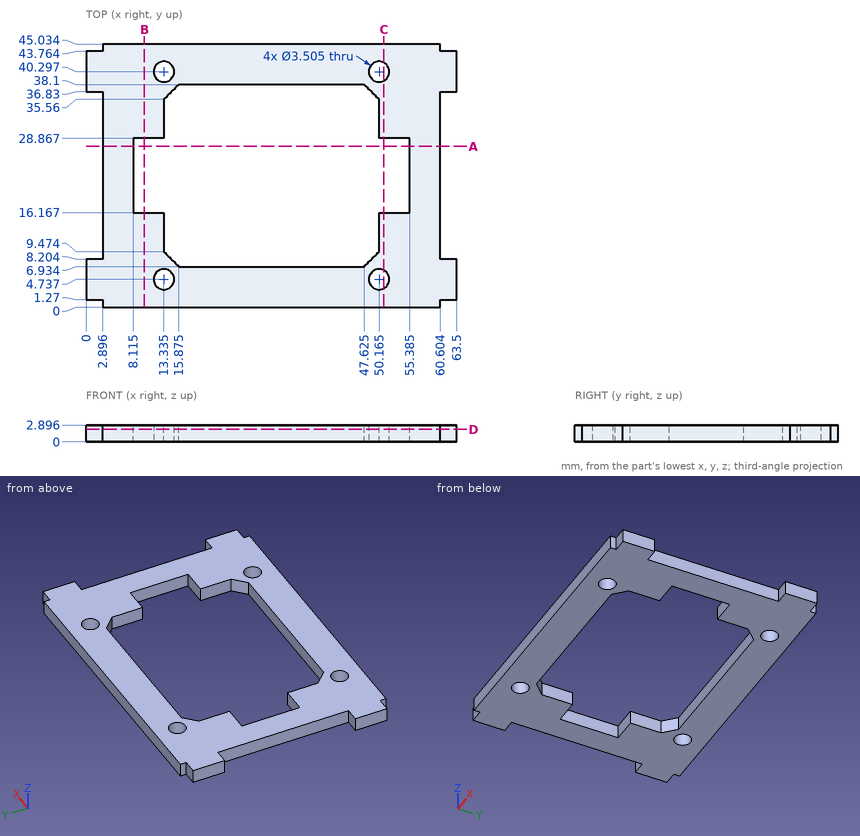
Job drawing, mm, ordinate dimensions from the low corner. One solid piece. Give positions to 0.01 mm unless a question says otherwise; leave off trailing zeros. Order: outer loops, then holes, each group sorted by start corner. A loop starts at its lowest first (then second) coordinate and runs counter-clockwise, first axis right, second up. Notation, with made-up numbers: M 63,4 L 89,4 A34 ccw 89,37 Z; hole C 25.25,26.5 d11. An arc over 180 degrees is marked long. Return JSON: item names as keys, results as strings.
Q1. Band-saw the part on D-D (z = 2.15). Count the separate pieces of the cut face and the enclosed holes in it, then the cut area to 3 significant figures.
Answer list:
{"separate pieces": "1", "enclosed holes": "5", "area": "1,370 mm^2"}
Q2. Band-saw the part on C-C (x = 51). Give the cut face in (y, z) (1 decimal).
Answer list:
{"outline": "M 0,0 L 3.2,0 L 3.2,2.9 L 0,2.9 Z; M 6.3,0 L 16.2,0 L 16.2,2.9 L 6.3,2.9 Z; M 28.9,0 L 38.8,0 L 38.8,2.9 L 28.9,2.9 Z; M 41.8,0 L 45,0 L 45,2.9 L 41.8,2.9 Z"}
Q3. Band-saw the part on A-A (y = 27.5). Give the cut face in (x, z) (1 decimal).
Answer list:
{"outline": "M 2.9,0 L 8.1,0 L 8.1,2.9 L 2.9,2.9 Z; M 55.4,0 L 60.6,0 L 60.6,2.9 L 55.4,2.9 Z"}
Q4. Band-saw the part on B-B (x = 10). Give the cut face in (y, z) (1 decimal).
Answer list:
{"outline": "M 0,0 L 16.2,0 L 16.2,2.9 L 0,2.9 Z; M 28.9,0 L 45,0 L 45,2.9 L 28.9,2.9 Z"}
Q5. Wall check: probe 1 along X at (y, z) = (40.5, 0.8) (1 decimal); probe 2 along X at (y, z) = (13.5, 1.55) (1 decimal); probe 3 along X at (y, z) = (20, 1.3) (1 decimal). Give the ranges that are in metal, low to high. Write a range as from..to.
Answer list:
{"probe 1": "x = 0..11.6, 15.1..48.4, 51.9..63.5", "probe 2": "x = 2.9..13.3, 50.2..60.6", "probe 3": "x = 2.9..8.1, 55.4..60.6"}
Q6. Flat gauge pins, fed straight in: pin 1 (1.4 mm diameter, centred on x = 62.5, z = 1, fed in from -Y); pin 2 (1 mm diameter, centred on y = 44.5, z = 1, fed in from -X); pin 3 (1.4 mm diameter, centred on x = 1.5, z = 1.5, fed in from +Y). Where does each tip first touch, or does it go through?
Answer list:
{"pin 1": "stops at y = 1.27", "pin 2": "stops at x = 2.9", "pin 3": "stops at y = 43.76"}
